from build123d import *

# Parameters (mm, degrees)
CHAMFER_SIZE = 1


with BuildPart() as part:
    # Sketch_1 → Revolution (revolve)
    with BuildSketch(Plane.YZ):
        Polygon((0, 0), (-7.5, 0), (-7.5, 4.5), (-15, 4.5), (-15, 9.5), (-10, 9.5), (-10, 12.5), (0, 12.5), align=None)
    revolve(axis=Axis((0, 0, 0), (0, 0, 1)))

    # Chamfer
    chamfer_edges = [part.edges().sort_by_distance(p)[0] for p in [
        (0, 7.5, 0),
        (0, 10, 12.5),
    ]]
    chamfer(chamfer_edges, length=CHAMFER_SIZE)


solid = part.part
Geometry: final body of the model. Coordinates: model frame, mm. A direction names the side the tool comes from. Round coordinates to 2 decimals unless told otherwise and drop trailing zeros. Write each loop counter-clockwise with the first axis right and the second up, starting at its lowest first coordinate (ties: lowest second). Pieces come first, ordered by that corner, then holes. Notation, with made-up numbers: M 75,-40 L 118,-40 A17 ccw 118,-19 Z; hole C 49,-27 d9. An arc over 180 degrees is marked long. Write item = value, one per line.
Item 1: Section query A-A on x = 0. Return loops of the section in (y, z), then the cut area to 4 significant figures.
Findings:
outline = M -15,4.5 L -7.5,4.5 L -7.5,1 L -6.5,0 L 6.5,0 L 7.5,1 L 7.5,4.5 L 15,4.5 L 15,9.5 L 10,9.5 L 10,11.5 L 9,12.5 L -9,12.5 L -10,11.5 L -10,9.5 L -15,9.5 Z
area = 275.5 mm^2
Item 2: Pin query (flat end, axial travel): P1, Ø5, axis at x = 10, y = 12, coming from the +Z side; P2, Ø5, axis at y = 7, z = 7, coming from the +X side; P3, Ø10, axis at x = -8.5, y = -10.5, coming from the -Z side. Return the tip coordinate at first contact, or that it passes through.
Findings:
P1 = 9.5
P2 = 14.31
P3 = 4.5
Item 3: Access query for faces 1 (the face through (-9.76, 2.17, 10.51)), 2 (the face through (0.33, 7.493, 2.774)), 3 (the face through (0.66, 14.985, 7.035)). Directions: +Z, -Z, +X, -X, +Y, -Y. A direction counts if a zero-diameter tool reaches every point of the face in a straight line with its end or side. Return the directions, or none.
Findings:
face_1 = +Z
face_2 = -Z
face_3 = +Z, -Z
Item 4: Section query D-D on z = 1.75. Return loops of the section in (x, y), then the cut area to 3 significant figures.
Findings:
outline = C 0,0 d15
area = 177 mm^2
Item 5: Section query C-C on z = 6. Return loops of the section in (x, y), then the cut area to 3 significant figures.
Findings:
outline = C 0,0 d30
area = 707 mm^2
Item 6: Material intervals for line 1 along Z through (x, y) = (-12, -3.5); line 2 along Z through (x, y) = (8, 3); line 3 along X through (y, z) = (9, 5), sorted ascending. Write a range as [from, to].
Findings:
line_1 = [4.5, 9.5]
line_2 = [4.5, 12.5]
line_3 = [-12, 12]
